Part model, mm, in its own coordinate system. Face numbers are marked on the shaded views. A direction names the side the tool comes from. Round coordinates to 2 decimals unless told otherwise and drop trailing zeros. Order: outer loops, then holes, each group sorted by start corner. A loop starts at its lowest first (then second) coordinate and runs counter-clockwise, first axis right, second up. Notation, with made-up numbers: (-16.5, 59) - (17.5, 59) arc R9 cw to (17.5, 65) - close; hole circle Ø10 at (-20, 60.25). An arc over 180 degrees is marked (long way). Return JSON: item names as keys, results as strings. Group by question number.
Item 1: Saw through at A-A on y = -18.5. List the corners of the cut face in (x, z).
Item 2: Tool access for the marked faces 1 and 2: list every direction of +Z, -Z, +X, -X, +Y, -Y with a clear straight run to the whole face (end or side of a thin tool).
Item 3: Two-plate mould, pull along X, no slides. Class the marked faces 3, 4 and 5: released by +X, released by -X, zero draft, split by the parting line, or undercut.
Item 4: Drop flat-ended pins along their axis: pin 1 (15 mm diameter, centred on x = 24.5, z = -21.5, fed in from -Y); pin 2 (2 mm diameter, centred on y = -3.5, z = -0.5, fed in from -X). Give the stop position or say it passes through.
Item 5: Saw through at C-C on x = -44.5. List the corners of the cut face in (y, z), and give its area (3 significant figures).
Item 6: Saw through at D-D on z = -11.5. List the corners of the cut face in (x, y).
Item 7: Saw through at B-B on z = 21. List the corners of the cut face in (x, y), and give its area (3 significant figures).
Item 8: Probe probe 1 along X at (y, z) = (-23.5, 23.5); probe 2 along Z at (x, y) = (-44, -14.5); probe 3 along X at (y, z) = (-9, -24). List the from-to ranges inside material, lowest first.
```python
from build123d import *

# Parameters (mm, degrees)
F0_W        = 127
F0_H        = 76.2
F1_DEPTH    = 30.48
F2_W        = 56.4744591247
F2_H        = 29.9161975272
F2_W_2      = 54.3375890702
F2_H_2      = 29.3056648225
F2_W_3      = 57.0849904325
F2_H_3      = 29.6109346673
F2_W_4      = 55.8639247902
F2_H_4      = 31.1372692231
F3_DEPTH    = 25.4
F4_T1_DEPTH = 152.4
F4_T3_DEPTH = 101.6


# Not quite as in the source:
# - a fillet or chamfer that OpenCascade refuses, or shapes differently, is made with other operations: its cross-section is extruded or revolved along the edge and cut away or added


with BuildPart() as f1:
    # F0 (on Front) → F1 (new body)
    with BuildSketch(Plane.XZ):
        Rectangle(F0_W, F0_H)
    extrude(amount=F1_DEPTH)

    # F2 (on face) → F3 (cut)
    with BuildSketch(Plane.XZ.offset(30.48)):
        with Locations((-31.5951720113, 19.2318481859)):
            Rectangle(F2_W, F2_H)
        with Locations((31.1372699216, 19.23184935)):
            Rectangle(F2_W_2, F2_H_2)
        with Locations((31.9004367338, -19.0792032517)):
            Rectangle(F2_W_3, F2_H_3)
        with Locations((-31.5951702651, -18.6213011621)):
            Rectangle(F2_W_4, F2_H_4)
    extrude(amount=-F3_DEPTH, mode=Mode.SUBTRACT)

    # F4: fillet of radius 5.08 on 8 edges, made by hand

    # F4_s2 → F4_t1 (cut)
    with BuildSketch(Plane.YZ.offset(-76.2)):
        with BuildLine():
            ThreePointArc((-25.4, -38.1), (-28.9921024484, -36.6121024484), (-30.48, -33.02))
            Line((-30.48, -33.02), (-30.48, -38.1))
            Line((-30.48, -38.1), (-25.4, -38.1))
        make_face()
        with BuildLine():
            ThreePointArc((-25.4, 38.1), (-28.9921024484, 36.6121024484), (-30.48, 33.02))
            Line((-30.48, 33.02), (-30.48, 38.1))
            Line((-30.48, 38.1), (-25.4, 38.1))
        make_face()
        with BuildLine():
            ThreePointArc((-5.08, -38.1), (-1.4878975516, -36.6121024484), (0, -33.02))
            Line((0, -33.02), (0, -38.1))
            Line((0, -38.1), (-5.08, -38.1))
        make_face()
        with BuildLine():
            ThreePointArc((-5.08, 38.1), (-1.4878975516, 36.6121024484), (0, 33.02))
            Line((0, 33.02), (0, 38.1))
            Line((0, 38.1), (-5.08, 38.1))
        make_face()
    extrude(amount=F4_T1_DEPTH, mode=Mode.SUBTRACT)

    # F4_s4 → F4_t3 (cut)
    with BuildSketch(Plane.XY.offset(-50.8)):
        with BuildLine():
            ThreePointArc((-58.42, -30.48), (-62.0121024484, -28.9921024484), (-63.5, -25.4))
            Line((-63.5, -25.4), (-63.5, -30.48))
            Line((-63.5, -30.48), (-58.42, -30.48))
        make_face()
        with BuildLine():
            ThreePointArc((63.5, -25.4), (62.0121024484, -28.9921024484), (58.42, -30.48))
            Line((58.42, -30.48), (63.5, -30.48))
            Line((63.5, -30.48), (63.5, -25.4))
        make_face()
        with BuildLine():
            ThreePointArc((-58.42, 0), (-62.0121024484, -1.4878975516), (-63.5, -5.08))
            Line((-63.5, -5.08), (-63.5, 0))
            Line((-63.5, 0), (-58.42, 0))
        make_face()
        with BuildLine():
            ThreePointArc((63.5, -5.08), (62.0121024484, -1.4878975516), (58.42, 0))
            Line((58.42, 0), (63.5, 0))
            Line((63.5, 0), (63.5, -5.08))
        make_face()
    extrude(amount=F4_T3_DEPTH, mode=Mode.SUBTRACT)


solid = f1.part
```
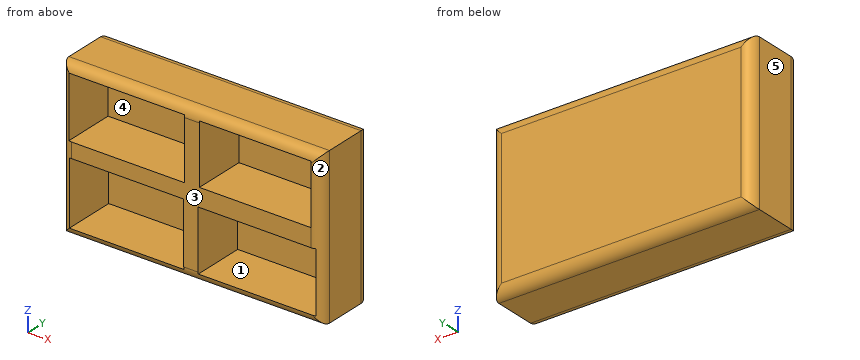
Filled in:
{
 "1": {"outline": "(-63.5, -38.1) - (63.5, -38.1) - (63.5, 38.1) - (-63.5, 38.1) - close; hole (-59.83, 4.27) - (-3.36, 4.27) - (-3.36, 34.19) - (-59.83, 34.19) - close; hole (-59.53, -34.19) - (-3.66, -34.19) - (-3.66, -3.05) - (-59.53, -3.05) - close; hole (3.36, -33.88) - (60.44, -33.88) - (60.44, -4.27) - (3.36, -4.27) - close; hole (3.97, 4.58) - (58.31, 4.58) - (58.31, 33.88) - (3.97, 33.88) - close"},
 "2": {"face 1": "-Y", "face 2": "+Z, -Z, +X, -Y"},
 "3": {"face 3": "zero draft", "face 4": "undercut", "face 5": "released by -X"},
 "4": {"pin 1": "stops at y = -5.08", "pin 2": "stops at x = -63.47"},
 "5": {"outline": "(-30.48, -3.05) - (-5.08, -3.05) - (-5.08, -34.19) - (-30.34, -34.19) arc R5.08 ccw to (-25.4, -38.1) - (-5.08, -38.1) arc R5.08 ccw to (0, -33.02) - (0, 33.02) arc R5.08 ccw to (-5.08, 38.1) - (-25.4, 38.1) arc R5.08 ccw to (-30.34, 34.19) - (-5.08, 34.19) - (-5.08, 4.27) - (-30.48, 4.27) - close", "area": "750 mm^2"},
 "6": {"outline": "(-63.5, -25.4) arc R5.08 ccw to (-59.53, -30.36) - (-59.53, -5.08) - (-3.66, -5.08) - (-3.66, -30.48) - (3.36, -30.48) - (3.36, -5.08) - (60.44, -5.08) - (60.44, -30.06) arc R5.08 ccw to (63.5, -25.4) - (63.5, -5.08) arc R5.08 ccw to (58.42, 0) - (-58.42, 0) arc R5.08 ccw to (-63.5, -5.08) - close"},
 "7": {"outline": "(-63.5, -25.4) arc R5.08 ccw to (-59.83, -30.28) - (-59.83, -5.08) - (-3.36, -5.08) - (-3.36, -30.48) - (3.97, -30.48) - (3.97, -5.08) - (58.31, -5.08) - (58.31, -30.48) - (58.42, -30.48) arc R5.08 ccw to (63.5, -25.4) - (63.5, -5.08) arc R5.08 ccw to (58.42, 0) - (-58.42, 0) arc R5.08 ccw to (-63.5, -5.08) - close", "area": "1,030 mm^2"},
 "8": {"probe 1": "x = -63.5 to -59.83, -3.36 to 3.97, 58.31 to 63.5", "probe 2": "z = -38.1 to -34.19, -3.05 to 4.27, 34.19 to 38.1", "probe 3": "x = -63.5 to -59.53, -3.66 to 3.36, 60.44 to 63.5"}
}
